Source: CAD feature listing. Evaluate the final solid. Frame: model axes, mm. Give positions to 0.01 mm unless a question says otherwise; leave off trailing zeros. Order: outer loops, then holes, each group sorted by start corner. A loop starts at its lowest first (then second) coordinate and runs counter-clockwise, first axis right, second up.
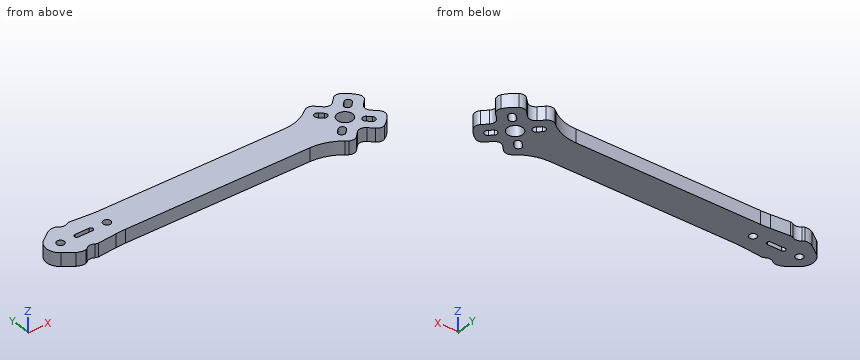
from build123d import *

# Parameters (mm, degrees)
SKETCH1_R                = 3.5
BOSS_EXTRUDE1_DEPTH      = 6
M3_CLEARANCE_HOLE1_D     = 3.4
M3_CLEARANCE_HOLE1_DEPTH = 6


with BuildPart() as part:
    # Sketch1 → Boss-Extrude1 (new body)
    with BuildSketch(Plane.XY):
        with BuildLine():
            Line((-118.078026422, -8.43859944), (-109.524525727, -7.690265095))
            ThreePointArc((-109.524525727, -7.690265095), (-107.347707958, -7.547588921), (-105.16673859, -7.5))
            Line((-105.16673859, -7.5), (-21.650635095, -7.5))
            ThreePointArc((-21.650635095, -7.5), (-15.104098388, -8.60177635), (-9.278843612, -11.785714286))
            ThreePointArc((-9.278843612, -11.785714286), (-8.704608747, -12.215964414), (-8.110455382, -12.618261112))
            ThreePointArc((-8.110455382, -12.618261112), (-6.167778591, -13.077430507), (-4.367043962, -12.215929233))
            Line((-4.367043962, -12.215929233), (-2.121320344, -9.970205615))
            ThreePointArc((-2.121320344, -9.970205615), (0, -9.091525958), (2.121320344, -9.970205615))
            Line((2.121320344, -9.970205615), (4.367043962, -12.215929233))
            ThreePointArc((4.367043962, -12.215929233), (6.167778591, -13.077430507), (8.110455382, -12.618261112))
            ThreePointArc((8.110455382, -12.618261112), (10.606601718, -10.606601718), (12.618261112, -8.110455382))
            ThreePointArc((12.618261112, -8.110455382), (13.077430507, -6.167778591), (12.215929233, -4.367043962))
            Line((12.215929233, -4.367043962), (9.970205615, -2.121320344))
            ThreePointArc((9.970205615, -2.121320344), (9.091525958, 0), (9.970205615, 2.121320344))
            Line((9.970205615, 2.121320344), (12.215929233, 4.367043962))
            ThreePointArc((12.215929233, 4.367043962), (13.077430507, 6.167778591), (12.618261112, 8.110455382))
            ThreePointArc((12.618261112, 8.110455382), (10.606601718, 10.606601718), (8.110455382, 12.618261112))
            ThreePointArc((8.110455382, 12.618261112), (6.167778591, 13.077430507), (4.367043962, 12.215929233))
            Line((4.367043962, 12.215929233), (2.121320344, 9.970205615))
            ThreePointArc((2.121320344, 9.970205615), (0, 9.091525958), (-2.121320344, 9.970205615))
            Line((-2.121320344, 9.970205615), (-4.367043962, 12.215929233))
            ThreePointArc((-4.367043962, 12.215929233), (-6.167778591, 13.077430507), (-8.110455382, 12.618261112))
            ThreePointArc((-8.110455382, 12.618261112), (-8.704608747, 12.215964414), (-9.278843612, 11.785714286))
            ThreePointArc((-9.278843612, 11.785714286), (-15.104098388, 8.60177635), (-21.650635095, 7.5))
            Line((-21.650635095, 7.5), (-105.16673859, 7.5))
            ThreePointArc((-105.16673859, 7.5), (-107.347707958, 7.547588921), (-109.524525727, 7.690265095))
            Line((-109.524525727, 7.690265095), (-118.078026422, 8.43859944))
            ThreePointArc((-118.078026422, 8.43859944), (-118.763989135, 8.379655937), (-119.389318724, 8.091589824))
            ThreePointArc((-119.389318724, 8.091589824), (-121.346764731, 7.570260106), (-123.189327607, 8.411890421))
            ThreePointArc((-123.189327607, 8.411890421), (-123.647802273, 8.746502417), (-124.181815085, 8.938842024))
            ThreePointArc((-124.181815085, 8.938842024), (-126.232348099, 8.932309996), (-128.107820511, 8.103255389))
            Line((-128.107820511, 8.103255389), (-132.322652835, 5.076759373))
            ThreePointArc((-132.322652835, 5.076759373), (-134.927242807, 0), (-132.322652835, -5.076759373))
            Line((-132.322652835, -5.076759373), (-128.107820511, -8.103255389))
            ThreePointArc((-128.107820511, -8.103255389), (-126.232348099, -8.932309996), (-124.181815085, -8.938842024))
            ThreePointArc((-124.181815085, -8.938842024), (-123.647802273, -8.746502417), (-123.189327607, -8.411890421))
            ThreePointArc((-123.189327607, -8.411890421), (-121.346764731, -7.570260106), (-119.389318724, -8.091589824))
            ThreePointArc((-119.389318724, -8.091589824), (-118.763989135, -8.379655937), (-118.078026422, -8.43859944))
        make_face()
        Circle(SKETCH1_R, mode=Mode.SUBTRACT)
        with BuildLine():
            Line((7.954951288, 5.762920267), (6.470027048, 4.277996026))
            ThreePointArc((6.470027048, 4.277996026), (4.277996026, 4.277996026), (4.277996026, 6.470027048))
            Line((4.277996026, 6.470027048), (5.762920267, 7.954951288))
            ThreePointArc((5.762920267, 7.954951288), (7.954951288, 7.954951288), (7.954951288, 5.762920267))
        make_face(mode=Mode.SUBTRACT)
        with BuildLine():
            Line((-5.762920267, 7.954951288), (-4.277996026, 6.470027048))
            ThreePointArc((-4.277996026, 6.470027048), (-4.277996026, 4.277996026), (-6.470027048, 4.277996026))
            Line((-6.470027048, 4.277996026), (-7.954951288, 5.762920267))
            ThreePointArc((-7.954951288, 5.762920267), (-7.954951288, 7.954951288), (-5.762920267, 7.954951288))
        make_face(mode=Mode.SUBTRACT)
        with BuildLine():
            Line((5.762920267, -7.954951288), (4.277996026, -6.470027048))
            ThreePointArc((4.277996026, -6.470027048), (4.277996026, -4.277996026), (6.470027048, -4.277996026))
            Line((6.470027048, -4.277996026), (7.954951288, -5.762920267))
            ThreePointArc((7.954951288, -5.762920267), (7.954951288, -7.954951288), (5.762920267, -7.954951288))
        make_face(mode=Mode.SUBTRACT)
        with BuildLine():
            Line((-7.954951288, -5.762920267), (-6.470027048, -4.277996026))
            ThreePointArc((-6.470027048, -4.277996026), (-4.277996026, -4.277996026), (-4.277996026, -6.470027048))
            Line((-4.277996026, -6.470027048), (-5.762920267, -7.954951288))
            ThreePointArc((-5.762920267, -7.954951288), (-7.954951288, -7.954951288), (-7.954951288, -5.762920267))
        make_face(mode=Mode.SUBTRACT)
        with BuildLine():
            Line((-121.427242807, 1), (-114.927242807, 1))
            ThreePointArc((-114.927242807, 1), (-113.927242807, 0), (-114.927242807, -1))
            Line((-114.927242807, -1), (-121.427242807, -1))
            ThreePointArc((-121.427242807, -1), (-122.427242807, 0), (-121.427242807, 1))
        make_face(mode=Mode.SUBTRACT)
    extrude(amount=BOSS_EXTRUDE1_DEPTH)

    # M3 Clearance Hole1
    with Locations(Plane.XY.offset(6)):
        with Locations((-107.677242807, 0), (-128.677242807, 0)):
            Hole(M3_CLEARANCE_HOLE1_D / 2, depth=M3_CLEARANCE_HOLE1_DEPTH)


solid = part.part
1) Section query C-C on z = 2.25. State how many separate pieces and enclosed holes the cut face has, and give its area (3 significant figures).
Checks:
separate pieces: 1
enclosed holes: 8
area: 2,270 mm2
2) Section query B-B on x = -53.5. Output: boundary loops of the cut face in (y, z), and give its area (3 significant figures).
Checks:
outline: (-7.5, 0) - (7.5, 0) - (7.5, 6) - (-7.5, 6) - close
area: 90.0 mm2
3) First-contact query: pin 1 Ø5.5 at (x, y) = (0, 0) entering from -Z; pin 2 Ø3 at (x, z) = (-101.5, 2.5) entering from +Y; pin 3 Ø1.8 at (x, z) = (-118, 3) entering from +Y. Flat tips, straight axial feed; report the tip coordinate or a pass-through.
Checks:
pin 1: passes through
pin 2: stops at y = 7.5
pin 3: stops at y = 8.45
4) Ray query, L1, parallel to X at y = 1.25, z = 5.2; L2, parallel to X at y = -0.75, z = 0.6; L3, parallel to Y at x = 0, z = 2.5. Return the intervals inside material, ascending.
Checks:
L1: x = -134.8 to -129.83, -127.53 to -108.83, -106.53 to -3.27, 3.27 to 9.36
L2: x = -134.88 to -130.2, -127.15 to -122.09, -114.27 to -109.2, -106.15 to -3.42, 3.42 to 9.19
L3: y = -9.09 to -3.5, 3.5 to 9.09
5) Section query D-D on x = -20. Output: boundary loops of the cut face in (y, z).
Checks:
outline: (-7.57, 0) - (7.57, 0) - (7.57, 6) - (-7.57, 6) - close
6) Section query A-A on x = 0. Output: boundary loops of the cut face in (y, z), and give its area (3 significant figures).
Checks:
outline: (-9.09, 0) - (-3.5, 0) - (-3.5, 6) - (-9.09, 6) - close; (3.5, 0) - (9.09, 0) - (9.09, 6) - (3.5, 6) - close
area: 67.1 mm2
